Could you check a few things on this model? Use its own coordinates, in mm. Face numbers are marked on the shaded views. A direction names the side the tool comes from. Give positions to 0.01 mm unless a question says otherwise; leave off trailing zeros. Write each loop counter-clockwise with the first axis right and the second up, starting at its lowest first coordinate (ties: lowest second). Pieces come first, ordered by that corner, then holes. Notation, with made-up numbers: (-22, -5) - (21, -5) arc R21 cw to (21, 15) - close; hole circle Ø10 at (-31, -28). An arc over 180 degrees is marked (long way). Answer as CSV lines item,"result". Start each with the question number.
Q1. Imagine slicing it at A-A on y = 6.35. List the corners of the cut face in (x, z) for me, and give its area (3 significant figures).
Q2. Imagine slicing it at D-D on y = 1. List the corners of the cut face in (x, z) for me (3 decimals).
Q3. Imagine slicing it at C-C on z = -2. List the corners of the cut face in (x, y) for me, and give its area (3 significant figures).
Q4. Will these pins go through, and if not, where does the flat tip stop? pin 1 Ø1.8 at (x, y) = (34.544, 6.35) entering from -Z; pin 2 Ø2 at (y, z) = (7.5, 1) entering from +X; pin 3 Ø4 at (x, y) = (67.056, 6.35) entering from +Z; pin 4 Ø4 at (x, z) = (23.5, -4.5) entering from +Y.
Q5. Imagine slicing it at B-B on x = 16. List the corners of the cut face in (y, z) for me, and give its area (3 significant figures).
Q6. If I drill on line 1 along X through (y, z) = (6.35, 1.7); line 2 along Z through (x, y) = (82.5, 2.25); line 3 along Z through (x, y) = (40.5, 5.25), over which ranges is the centre line in solid material (lowest first)?
Q7. On a 3-axis mill with a long thin cutter (end or side, diameter ignored), from which of +Z, -Z, +X, -X, +Y, -Y can I reach the whole of each face in a straight line? I mean the marked faces 1 and 2. Say none if no direction works.
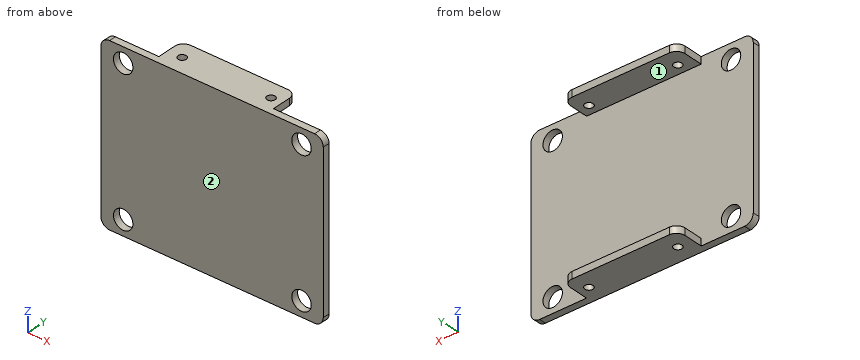
Autodesk Inventor part; units mm, degrees
ref_plane "YZ Plane" through (0, 0, 0) normal (1, 0, 0) x (0, 1, 0)
ref_plane "XZ Plane" through (0, 0, 0) normal (0, 1, 0) x (-1, 0, 0)
ref_plane "XY Plane" through (0, 0, 0) normal (0, 0, 1) x (1, 0, 0)
sketch "Sketch1" plane through (0, 0, 0) normal (0, 0, 1) x (1, 0, 0)
  line L0 (0, 0) -> (101.6, 0)
  line L1 (101.6, 0) -> (101.6, 12.7)
  line L2 (101.6, 12.7) -> (0, 12.7)
  line L3 (0, 12.7) -> (0, 0)
  dimension "d0" = 101.6
  dimension "d1" = 12.7
extrude "Extrusion1" add sketch "Sketch1" along normal blind 2.54
sketch "Sketch2" plane through (0, 0, 0) normal (0, 0, -1) x (-1, 0, 0)
  line L0 (-101.6, 0) -> (-101.6, 12.7)
  line L1 (0, 0) -> (-101.6, 0)
  line L2 (-101.6, 0) -> (-101.6, 2.54)
  line L3 (-101.6, 2.54) -> (0, 2.54)
  line L4 (0, 2.54) -> (0, 0)
  dimension "d4" = 2.54
extrude "Extrusion2" add sketch "Sketch2" along normal blind 58.42
sketch "Sketch3" plane through (0, 0, -58.42) normal (0, 0, -1) x (-1, 0, 0)
  line L0 (-101.6, 12.7) -> (0, 12.7)
  line L1 (0, 0) -> (-101.6, 0)
  line L2 (-101.6, 0) -> (-101.6, 12.7)
  line L3 (-101.6, 12.7) -> (0, 12.7)
  line L4 (0, 12.7) -> (0, 0)
  dimension "d19" = 101.6
extrude "Extrusion3" add sketch "Sketch3" along normal blind 2.54
sketch "Sketch4" plane through (0, 0, 2.54) normal (0, 0, 1) x (1, 0, 0)
  line L0 (101.6, 12.7) -> (0, 12.7)
  line L1 (101.6, 0) -> (101.6, 12.7)
  point P0 (0, 0)
  point P1 (67.056, 6.35)
  point P2 (34.544, 6.35)
  dimension "d9" = 32.512
  dimension "d10" = 6.35
  dimension "d11" = 6.35
  dimension "d20" = 34.544
hole "Hole1" at (67.056, 6.35, 2.54) at (34.544, 6.35, 2.54) direction (0, 0, -1) diameter 2.9972 end through all
sketch "Sketch5" plane through (0, 0, 2.54) normal (0, -1, 0) x (1, 0, 0)
  line L0 (101.6, -63.5) -> (101.6, 0)
  line L1 (0, 0) -> (101.6, 0)
  line L2 (0, 0) -> (0, -63.5)
  line L3 (101.6, -63.5) -> (0, -63.5)
  point P0 (0, -2.54)
  point P1 (83.4898, -5.5372)
  point P2 (18.288, -5.5372)
  point P3 (18.288, -57.9628)
  point P4 (83.4898, -57.9628)
  dimension "d21" = 18.1102
  dimension "d22" = 5.5372
  dimension "d23" = 5.5372
  dimension "d24" = 18.288
  dimension "d25" = 18.1102
  dimension "d26" = 5.5372
  dimension "d27" = 5.5372
  dimension "d28" = 18.288
hole "Hole2" at (83.4898, 0, -2.9972) at (18.288, 0, -2.9972) at (18.288, 0, -55.4228) at (83.4898, 0, -55.4228) direction (0, 1, 0) diameter 7.112 end through all
sketch "Sketch6" plane through (0, 0, 2.54) normal (0, 0, 1) x (1, 0, 0)
  circle A0 centre (34.544, 6.35) radius 1.4986
  line L0 (33.0454, 6.35) -> (18.288, 6.35)
  circle A1 centre (67.056, 6.35) radius 1.4986
  line L1 (68.5546, 6.35) -> (83.4898, 6.35)
  line L2 (68.5546, 6.35) -> (83.4898, 6.35) construction
  point P0 (0, 0)
  dimension "d36" = 14.7574
  dimension "d37" = 14.9352
  dimension "d38" = 0
sketch "Sketch8" plane through (0, 0, -60.96) normal (0, 0, -1) x (-1, 0, 0)
  line L0 (0, 0) -> (0, 2.54)
  line L1 (0, 0) -> (0, 12.7)
  line L2 (0, 12.7) -> (-29.211, 12.7)
  line L3 (-29.211, 12.7) -> (-29.211, 2.54)
  line L4 (-29.211, 2.54) -> (0, 2.54)
  line L5 (0, 2.54) -> (0, 12.7)
  dimension "d39" = 2.54
  dimension "d51" = 29.211
extrude "Extrusion4" cut sketch "Sketch8" against normal through all
sketch "Sketch9" plane through (0, 0, 2.54) normal (0, -1, 0) x (1, 0, 0)
  line L0 (0, -63.5) -> (29.211, -63.5)
  line L1 (0, 0) -> (10.16, 0)
  line L2 (10.16, 0) -> (10.16, -63.5)
  line L3 (10.16, -63.5) -> (0, -63.5)
  line L4 (0, -63.5) -> (0, 0)
  line L5 (101.6, -2.54) -> (101.6, 0)
  line L6 (29.211, -63.5) -> (101.6, -63.5)
  line L7 (101.6, 0) -> (91.44, 0)
  line L8 (91.44, 0) -> (91.44, -63.5)
  line L9 (91.44, -63.5) -> (101.6, -63.5)
  line L10 (101.6, -63.5) -> (101.6, 0)
  point P0 (0, -2.54)
  dimension "d42" = 10.16
  dimension "d43" = 10.16
extrude "Extrusion5" cut sketch "Sketch9" against normal blind 25.4
sketch "Sketch10" plane through (0, 0, 2.54) normal (0, 0, 1) x (1, 0, 0)
  line L0 (10.16, 0) -> (91.44, 0)
  line L1 (91.44, 0) -> (91.44, 2.54)
  line L2 (91.44, 12.7) -> (29.211, 12.7)
  line L3 (91.44, 2.54) -> (71.12, 2.54)
  line L4 (71.12, 2.54) -> (71.12, 12.7)
  line L5 (71.12, 12.7) -> (91.44, 12.7)
  line L6 (91.44, 12.7) -> (91.44, 2.54)
  point P0 (0, 0)
  dimension "d46" = 2.54
  dimension "d47" = 20.32
extrude "Extrusion6" cut sketch "Sketch10" against normal through all
fillet "Fillet1" radius 3.175 8 edges at (71.12, 12.7, 1.27) (29.211, 12.7, 1.27) (10.16, 1.27, -60.96) (10.16, 1.27, 2.54) (29.211, 12.7, -59.69) (71.12, 12.7, -59.69) (91.44, 1.27, -60.96) (91.44, 1.27, 2.54)
equation "\"d43\" = d42"
properties part number "track guide u channel"
Conclusion:
1,outline,"(29.21, -60.96) - (33.05, -60.96) - (33.05, -58.42) - (29.21, -58.42) - close; (29.21, 0) - (33.05, 0) - (33.05, 2.54) - (29.21, 2.54) - close; (36.04, -60.96) - (65.56, -60.96) - (65.56, -58.42) - (36.04, -58.42) - close; (36.04, 0) - (65.56, 0) - (65.56, 2.54) - (36.04, 2.54) - close; (68.55, -60.96) - (71.12, -60.96) - (71.12, -58.42) - (68.55, -58.42) - close; (68.55, 0) - (71.12, 0) - (71.12, 2.54) - (68.55, 2.54) - close"
1,area,"182 mm^2"
2,outline,"(10.16, -57.785) arc R3.175 ccw to (13.335, -60.96) - (88.265, -60.96) arc R3.175 ccw to (91.44, -57.785) - (91.44, -0.635) arc R3.175 ccw to (88.265, 2.54) - (13.335, 2.54) arc R3.175 ccw to (10.16, -0.635) - close; hole circle Ø7.112 at (18.288, -55.423); hole circle Ø7.112 at (18.288, -2.997); hole circle Ø7.112 at (83.49, -55.423); hole circle Ø7.112 at (83.49, -2.997)"
3,outline,"(10.16, 0) - (14.87, 0) - (14.87, 2.54) - (10.16, 2.54) - close; (21.7, 0) - (80.08, 0) - (80.08, 2.54) - (21.7, 2.54) - close; (86.9, 0) - (91.44, 0) - (91.44, 2.54) - (86.9, 2.54) - close"
3,area,"172 mm^2"
4,pin 1,"through"
4,pin 2,"x = 71.12"
4,pin 3,"z = 2.54"
4,pin 4,"y = 2.54"
5,outline,"(0, -60.96) - (2.54, -60.96) - (2.54, -58.14) - (0, -58.14) - close; (0, -52.7) - (2.54, -52.7) - (2.54, -5.72) - (0, -5.72) - close; (0, -0.28) - (2.54, -0.28) - (2.54, 2.54) - (0, 2.54) - close"
5,area,"134 mm^2"
6,line 1,"29.21 to 33.05, 36.04 to 65.56, 68.55 to 71.12"
6,line 2,"-60.96 to -58.84, -52.01 to -6.41, 0.42 to 2.54"
6,line 3,"-60.96 to -58.42, 0 to 2.54"
7,face 1,"+X, -X, +Y"
7,face 2,"+Z, -Z, +X, -X, -Y"
